Design review of the part shown in the three views and the two pictorial views. Dimensions are in mm from the part's minimum x, y and z. Give positions to 0.01 mm unless a question says otherwise; leave off trailing zeros. Loops run counter-clockwise (first coordinate to the right, second up) from the corner with the lowest first, then second, coordinate; pieces in that order, holes last. Notation, with made-up numbers: (-31, -24.75) -> (-18, -24.75) arc R28 ccw to (-18, 8.25) -> close; hole circle Ø10 at (85, 76.25). An arc over 180 degrees is marked (long way). One line per question, with ' | ' between items. Start each with the question number.
(1) Wall thickness on probe 1 along X at (y, z) = (107, 0.95); probe 2 along Y at (x, z) = (85, 1.8); probe 3 along Y at (x, z) = (12, 1.2): over which ranges is each line inside the solid? List them lowest first.
(2) Consider section B-B (x = 98). Write out the cut boundary in (y, z).
(3) Consider section C-C (z = 0.5). Write out the cut boundary in (x, y) (1 decimal), and give its area (3 significant figures).
(4) Consider section A-A (y = 52). Write out the cut boundary in (x, z).
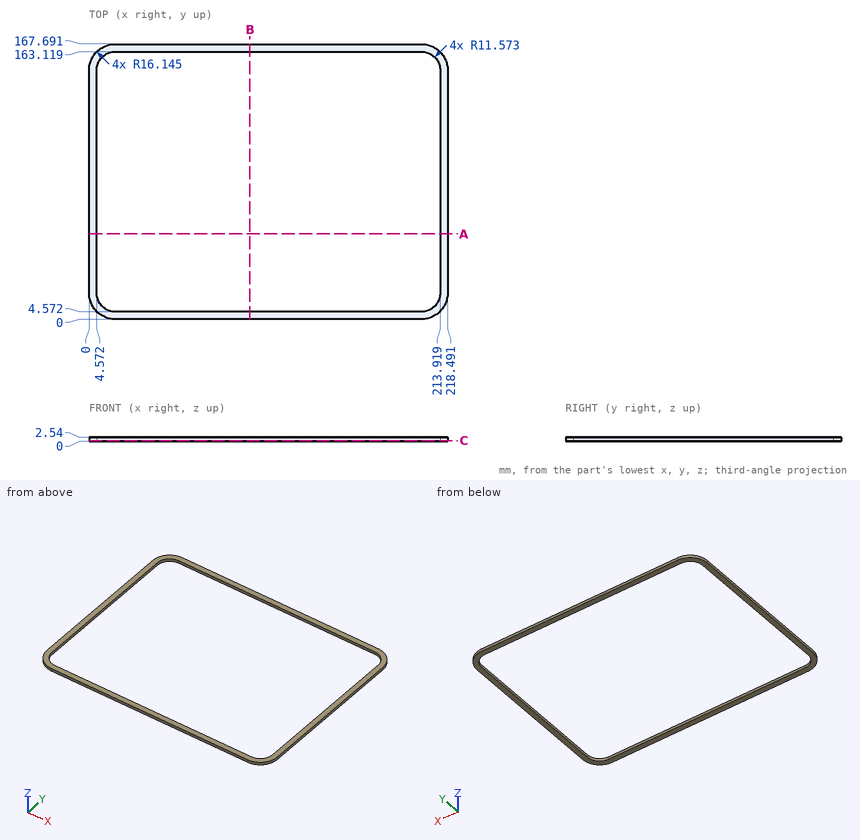
A:
1) probe 1: x = 0 to 4.57, 213.92 to 218.49 | probe 2: y = 0 to 4.57, 163.12 to 167.69 | probe 3: y = 0.54 to 5.34, 162.35 to 167.15
2) outline: (0, 0) -> (4.57, 0) -> (4.57, 2.54) -> (0, 2.54) -> close; (163.12, 0) -> (167.69, 0) -> (167.69, 2.54) -> (163.12, 2.54) -> close
3) outline: (0, 16.1) arc R16.1 ccw to (16.1, 0) -> (202.3, 0) arc R16.1 ccw to (218.5, 16.1) -> (218.5, 151.5) arc R16.1 ccw to (202.3, 167.7) -> (16.1, 167.7) arc R16.1 ccw to (0, 151.5) -> close; hole (4.6, 16.1) arc R11.6 ccw to (16.1, 4.6) -> (202.3, 4.6) arc R11.6 ccw to (213.9, 16.1) -> (213.9, 151.5) arc R11.6 ccw to (202.3, 163.1) -> (16.1, 163.1) arc R11.6 ccw to (4.6, 151.5) -> close | area: 3,340 mm^2
4) outline: (0, 0) -> (4.57, 0) -> (4.57, 2.54) -> (0, 2.54) -> close; (213.92, 0) -> (218.49, 0) -> (218.49, 2.54) -> (213.92, 2.54) -> close
